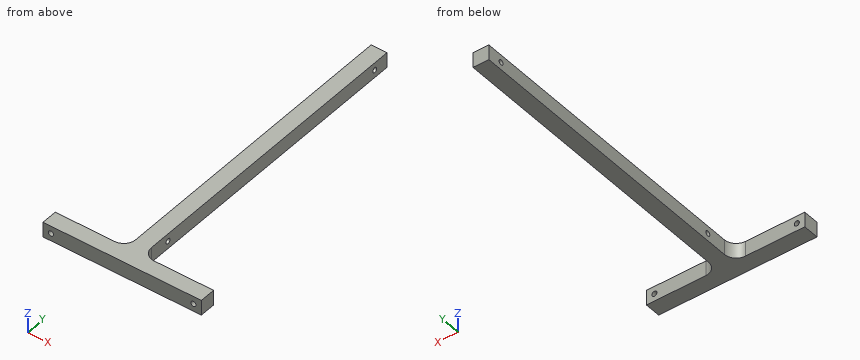
from build123d import *

# Parameters (mm, degrees)
BOSS_EXTRUDE1_DEPTH = 9.525
FILLET1_R           = 7.5
SKETCH2_R           = 1.625
CUT_EXTRUDE1_DEPTH  = 11
SKETCH3_R           = 1.625
CUT_EXTRUDE2_DEPTH  = 56


with BuildPart() as part:
    # Sketch1 → Boss-Extrude1 (new body)
    with BuildSketch(Plane.XY):
        Polygon((-50, 0), (50, 0), (50, 10), (5, 10), (5, 210), (-5, 210), (-5, 10), (-50, 10), align=None)
    extrude(amount=BOSS_EXTRUDE1_DEPTH)

    # Fillet1
    fillet1_edges = [part.edges().sort_by_distance(p)[0] for p in [
        (-5, 10, 4.7625),
        (5, 10, 4.7625),
    ]]
    fillet(fillet1_edges, radius=FILLET1_R)

    # Sketch2 → Cut-Extrude1 (cut, through all)
    with BuildSketch(Plane(origin=(0, 10, 0), x_dir=(1, 0, 0), z_dir=(0, 1, 0))):
        with Locations((-45, -4.7625)):
            Circle(SKETCH2_R)
        with Locations((45, -4.7625)):
            Circle(SKETCH2_R)
    extrude(amount=-CUT_EXTRUDE1_DEPTH, mode=Mode.SUBTRACT)

    # Sketch3 → Cut-Extrude2 (cut, through all)
    with BuildSketch(Plane.ZY.offset(5)):
        with Locations((4.7625, 31)):
            Circle(SKETCH3_R)
        with Locations((4.7625, 200)):
            Circle(SKETCH3_R)
    extrude(amount=-CUT_EXTRUDE2_DEPTH, mode=Mode.SUBTRACT)


solid = part.part
Design review of the part built by this model. Coordinates are the model's own, in mm. Give positions to 0.01 mm unless a question says otherwise; leave off trailing zeros. Write each loop counter-clockwise with the first axis right and the second up, starting at its lowest first coordinate (ties: lowest second). Pieces come first, ordered by that corner, then holes. Notation, with made-up numbers: M 17.5,79 L 58.5,79 A36 ccw 58.5,116 Z; hole C 13,-6.75 d5. An arc over 180 degrees is marked long. Return JSON: item names as keys, results as strings. Group by question number.
Item 1: Take a section at A-A (x = 23). Give the boundary of the cut face in (y, z) (3 decimals), plus the area to 4 significant figures.
Item 2: Clearance check with flat-ended pins moving along their axes: pin 1 Ø1.5 at (x, z) = (-12, 3) entering from +Y; pin 2 Ø4 at (x, z) = (11, 2.5) entering from -Y; pin 3 Ø5 at (x, z) = (-29, 5.5) entering from +Y; pin 4 Ø1 at (y, z) = (143, 7.5) entering from -X. State where each tip first meets the part, or that it passes through.
Item 3: Take a section at B-B (y = 100.5). Give the boundary of the cut face in (x, z) (3 decimals), plus the area to 4 significant figures.
Item 4: Wall thickness on line 1 along Z through (x, y) = (-45, 5) (1 decimal); line 2 along Y through (x, z) = (25, 7.75); line 3 along X through (y, z) = (186.5, 4.5): over which ranges is each line inside the solid? List them lowest first.
Return value:
{
 "1": {"outline": "M 0,0 L 10,0 L 10,9.525 L 0,9.525 Z", "area": "95.25 mm2"},
 "2": {"pin 1": "stops at y = 10.1", "pin 2": "stops at y = 0", "pin 3": "stops at y = 10", "pin 4": "stops at x = -5"},
 "3": {"outline": "M -5,0 L 5,0 L 5,9.525 L -5,9.525 Z", "area": "95.25 mm2"},
 "4": {"line 1": "z = 0 to 3.1, 6.4 to 9.5", "line 2": "y = 0 to 10", "line 3": "x = -5 to 5"}
}
